```python
from build123d import *

# Parameters (mm, degrees)
BOSS_EXTRUDE1_DEPTH = 100
BOSS_EXTRUDE2_DEPTH = 31
BOSS_EXTRUDE3_DEPTH = 4
SKETCH4_R           = 4.5
CUT_EXTRUDE1_DEPTH  = 137.315809795
SKETCH3_4_R         = 5
BOSS_EXTRUDE4_DEPTH = 2


with BuildPart() as part:
    # Sketch1 → Boss-Extrude1 (new body)
    with BuildSketch(Plane.XY):
        Polygon((0, 0), (0, 13), (3, 13), (3, 3), (32, 3), (32, 13), (35, 13), (35, 0), align=None)
    extrude(amount=BOSS_EXTRUDE1_DEPTH)

    # Sketch2 → Boss-Extrude2 (add)
    with BuildSketch(Plane.XY.offset(100)):
        Polygon((3, 6), (3, 3), (32, 3), (32, 6), (35, 6), (35, 0), (0, 0), (0, 6), align=None)
    extrude(amount=BOSS_EXTRUDE2_DEPTH)

    # Sketch3 → Boss-Extrude3 (add)
    # profile 1 of 2: a face of its own
    with BuildSketch(Plane.XY.offset(131)):
        Polygon((0, 17), (0, 6), (3, 6), (3, 3), (32, 3), (32, 6), (35, 6), (35, 17), align=None)
        Polygon((21.108439182, 16.25), (24.716878365, 10), (21.108439182, 3.75), (13.891560818, 3.75), (10.283121635, 10), (13.891560818, 16.25), align=None, mode=Mode.SUBTRACT)
    # profile 2 of 2: a face of its own
    with BuildSketch(Plane.XY.offset(131)):
        Polygon((3, 3), (3, 6), (0, 6), (0, 0), (35, 0), (35, 6), (32, 6), (32, 3), align=None)
    extrude(amount=-BOSS_EXTRUDE3_DEPTH)

    # Sketch4 → Cut-Extrude1 (cut, through all)
    with BuildSketch(Plane(origin=(0, 3, 0), x_dir=(1, 0, 0), z_dir=(0, 1, 0))):
        with Locations(Location((17.5, -107, 0), (0, 0, 180))):
            Circle(SKETCH4_R)
        with Locations(Location((17.5, -26.075, 0), (0, 0, 180))):
            Circle(SKETCH4_R)
    extrude(amount=-CUT_EXTRUDE1_DEPTH, mode=Mode.SUBTRACT)

    # Sketch3_4 → Boss-Extrude4 (add)
    # profile 1 of 3: a face of its own
    with BuildSketch(Plane.XY.offset(131)):
        Polygon((0, 17), (0, 6), (3, 6), (3, 3), (32, 3), (32, 6), (35, 6), (35, 17), align=None)
        Polygon((21.108439182, 16.25), (24.716878365, 10), (21.108439182, 3.75), (13.891560818, 3.75), (10.283121635, 10), (13.891560818, 16.25), align=None, mode=Mode.SUBTRACT)
    # profile 2 of 3: a face of its own
    with BuildSketch(Plane.XY.offset(131)):
        Polygon((3, 3), (3, 6), (0, 6), (0, 0), (35, 0), (35, 6), (32, 6), (32, 3), align=None)
    # profile 3 of 3: a face of its own
    with BuildSketch(Plane.XY.offset(131)):
        Polygon((13.891560818, 3.75), (21.108439182, 3.75), (24.716878365, 10), (21.108439182, 16.25), (13.891560818, 16.25), (10.283121635, 10), align=None)
        with Locations((17.5, 10)):
            Circle(SKETCH3_4_R, mode=Mode.SUBTRACT)
    extrude(amount=BOSS_EXTRUDE4_DEPTH)


solid = part.part
```
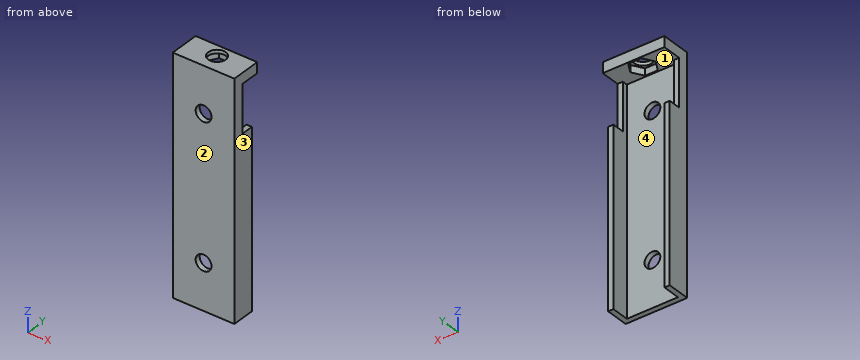
Check sheet for the modelled part. Datum: model origin and axes. Units: mm. Face numbers are marked on the shaded views. Give positions to 0.01 mm unless a question says otherwise; leave off trailing zeros. Order: outer loops, then holes, each group sorted by start corner. A loop starts at its lowest first (then second) coordinate and runs counter-clockwise, first axis right, second up. Notation, with made-up numbers: M 54.5,40 L 62.5,40 A21 ccw 62.5,63 Z; hole C 15.5,19.25 d2. An arc over 180 degrees is marked long. Answer in a Markdown table with one row per item.
1) Cross-section at A-A, the plane x = 17.5. Enter the section's corners in (y, z) (3 decimals), plus the area to 3 significant figures.
Filled sheet:
| item | result |
|---|---|
| outline | M 0,0 L 3,0 L 3,21.575 L 0,21.575 Z; M 0,30.575 L 3,30.575 L 3,102.5 L 0,102.5 Z; M 0,111.5 L 3,111.5 L 3,127 L 3.75,127 L 3.75,131 L 5,131 L 5,133 L 0,133 Z; M 15,131 L 16.25,131 L 16.25,127 L 17,127 L 17,133 L 15,133 Z |
| area | 359 mm2 |
2) Gauge pin test, flat ends, axial feed: P1, Ø1.5, axis at x = 7, z = 76, coming from the -Y side; P2, Ø1.5, axis at x = 33, z = 31, coming from the +Y side; P3, Ø5.5, axis at x = 17.5, z = 26.075, coming from the -Y side; P4, Ø4, axis at x = 27.5, z = 43, coming from the +Y side. Record the tip position at first contact, or that the pin passes through.
Filled sheet:
| item | result |
|---|---|
| P1 | stops at y = 0 |
| P2 | stops at y = 13 |
| P3 | passes through |
| P4 | stops at y = 3 |
3) Cross-section at D-D, the plane x = 8. Enter the section's corners in (y, z).
Filled sheet:
| item | result |
|---|---|
| outline | M 0,0 L 3,0 L 3,127 L 17,127 L 17,133 L 0,133 Z |
4) Cross-section at C-C, the plane z = 13. Enter the section's corners in (x, y).
Filled sheet:
| item | result |
|---|---|
| outline | M 0,0 L 35,0 L 35,13 L 32,13 L 32,3 L 3,3 L 3,13 L 0,13 Z |
5) Release check for a two-part mould opening along X. For the marked faces 1, 2, 3 and 4 record: +X half, -X half, draft (parallel to the pull), parting line (faces both ways), or undercut.
Filled sheet:
| item | result |
|---|---|
| face 1 | undercut |
| face 2 | draft |
| face 3 | +X half |
| face 4 | undercut |
6) Cross-section at B-B, the plane z = 107. Enter the section's corners in (x, y).
Filled sheet:
| item | result |
|---|---|
| outline | M 0,0 L 13,0 L 13,3 L 3,3 L 3,6 L 0,6 Z; M 22,0 L 35,0 L 35,6 L 32,6 L 32,3 L 22,3 Z |
7) Thickness scan on L1, parallel to X at y = 5.75, z = 13.5; L2, parallel to Y at x = 17.5, z = 131.6; L3, parallel to Z at x = 17.5, y = 0.6 (3 decimals). Record the ranges inside material, lowest first. Write a range as [from, to].
Filled sheet:
| item | result |
|---|---|
| L1 | x = [0, 3], [32, 35] |
| L2 | y = [0, 5], [15, 17] |
| L3 | z = [0, 21.575], [30.575, 102.5], [111.5, 133] |
